Input: part model. Units: mm. Frame: model coordinates. A direction names the side the tool comes from. Coordinates: 2 decimals unless noted, no trailing zeros. Loops run counter-clockwise (first coordinate to the right, second up) from the corner with the lowest first, then second, coordinate; pieces in that order, holes last.
Item 1: Section A-A on z = 14.5. Return loops of the section in (x, y), and give its area (3 significant figures).
Item 2: Contact query for a flat-ended pin moving along its axis: P1, Ø5, axis at x = 14.5, y = 23.5, coming from the +Z side. Output: stop coordinate, or through.
Item 3: Pull-direction query (Y, two-part tool) for faces 3 (the flat face through (57.5, -1, 15)), 4 (the cylindrical face through (-56.64, 44.1, 15.21)), 5 (the flat face through (-1, -42.5, 16)); classes: released by +Y, released by -Y, zero draft, split by the parting line, or undercut.
Item 4: Section B-B on y = 7. Return loops of the section in (x, z).
Item 5: Section C-C on x = 9. Return loops of the section in (y, z), and give its area (3 significant figures).
Item 6: Reachability of faces 1 (the flat face through (-55.5, -1, 16)), 2 (the flat face through (-1, 45, 15)) from +Z, -Z, +X, -X, +Y, -Y: full face, straight path, thin tool, end or side. Return the list, or none.
Item 7: Ray query, line 1 along X through (y, z) = (18, 11); line 2 along Y through (x, z) = (14.5, 28.25); line 3 along Z through (x, y) = (45, 14). Return the intervals inside material, ascending.
```python
from build123d import *

# Parameters (mm, degrees)
F0_W     = 115
F0_H     = 90
F1_DEPTH = 30
F3_W     = 111
F3_H     = 85
F4_DEPTH = 28
F5_R     = 3


# Not quite as in the source:
# - a feature names something its author has since deleted; it is built from what else it names


with BuildPart() as f1:
    # F0 (on Top) → F1 (new body)
    with BuildSketch(Plane.XY):
        Rectangle(F0_W, F0_H)
    extrude(amount=F1_DEPTH)

    # F3 (on offset) → F4 (cut)
    with BuildSketch(Plane.XY.offset(30)):
        Rectangle(F3_W, F3_H)
    extrude(amount=-F4_DEPTH, mode=Mode.SUBTRACT)

    # F5
    f5_edges = [f1.edges().sort_by_distance(p)[0] for p in [
        (-57.5, 45, 15),
        (57.5, 45, 15),
        (57.5, -45, 15),
        (-57.5, -45, 15),
    ]]
    fillet(f5_edges, radius=F5_R)


solid = f1.part
```
Results found:
1. outline: (-57.5, -42) arc R3 ccw to (-54.5, -45) - (54.5, -45) arc R3 ccw to (57.5, -42) - (57.5, 42) arc R3 ccw to (54.5, 45) - (-54.5, 45) arc R3 ccw to (-57.5, 42) - close; hole (-55.5, -42.5) - (55.5, -42.5) - (55.5, 42.5) - (-55.5, 42.5) - close
1. area: 907 mm2
2. P1: stops at z = 2
3. face 3: zero draft
3. face 4: released by +Y
3. face 5: undercut
4. outline: (-57.5, 0) - (57.5, 0) - (57.5, 30) - (55.5, 30) - (55.5, 2) - (-55.5, 2) - (-55.5, 30) - (-57.5, 30) - close
5. outline: (-45, 0) - (45, 0) - (45, 30) - (42.5, 30) - (42.5, 2) - (-42.5, 2) - (-42.5, 30) - (-45, 30) - close
5. area: 320 mm2
6. face 1: +Z
6. face 2: +Z, -Z, +X, -X, +Y
7. line 1: x = -57.5 to -55.5, 55.5 to 57.5
7. line 2: y = -45 to -42.5, 42.5 to 45
7. line 3: z = 0 to 2
